from build123d import *

# Parameters (mm, degrees)
F0_W     = 56.3871189952
F0_H     = 33.6253512651
F1_DEPTH = 2
F2_W     = 51.7
F2_H     = 11.2356165416
F3_DEPTH = 15.62
F4_W     = 51.7
F4_H     = 15.62
F5_DEPTH = 1.5


# Not quite as in the source:
# - a feature of the source that left no trace in its solid (it failed there, or was rolled back) is left out


with BuildPart() as f1:
    # F0 (on Top) → F1 (new body)
    with BuildSketch(Plane.XY):
        with Locations((-6.0005225241, 2.1580690518)):
            Rectangle(F0_W, F0_H)
    extrude(amount=F1_DEPTH)

    # F2 (on face) → F3 (join)
    with BuildSketch(Plane.XY.offset(2)):
        with Locations((-5.8556830972, -9.0367983099)):
            Rectangle(F2_W, F2_H)
    extrude(amount=F3_DEPTH)

    # F4 (on face) → F5 (join)
    with BuildSketch(Plane.XZ.offset(14.6546065807)):
        with Locations((-5.8556830972, 9.81)):
            Rectangle(F4_W, F4_H)
    extrude(amount=F5_DEPTH)


solid = f1.part
Verification items for the finished model (mm, model axes). A direction names the side the tool comes from. Coordinates: 2 decimals unless noted, no trailing zeros. Order: outer loops, then holes, each group sorted by start corner. A loop starts at its lowest first (then second) coordinate and runs counter-clockwise, first axis right, second up. Notation, with made-up numbers: M -27,-2.75 L 21,-2.75 A5 cw 21,5.25 Z; hole C 15,-17 d6. An arc over 180 degrees is marked long. One line per item, written item: value. Start each with the question number.
Item 1: Sectioned sample at A-A (y = -13.5). Enter the section's corners in (x, z), then the cut area to 3 significant figures.
Item 2: Gauge pin test, flat ends, axial feed: pin 1 (1 mm diameter, centred on y = -7, z = 9.5, fed in from -X); pin 2 (1.6 mm diameter, centred on x = -8, y = -15.5, fed in from -Z); pin 3 (2 mm diameter, centred on x = 9, z = 11.5, fed in from +Y). Record the tip position at first contact, or that the pin passes through.
Item 3: Access from +Z, -Z, +X, -X, +Y, -Y to the whole of each face (thin tool, end or side, straight path). Record for faces 1 (the flat face through (19.994, -10, 10)), 2 (the flat face through (-6, -14.655, 1)), 3 (the flat face through (-31.706, -10, 10)), 4 (the flat face through (-6, -3.419, 10)), 5 (the flat face through (-34.194, 2, 1)).
Item 4: Sectioned sample at D-D (y = 4.5). Enter the section's corners in (x, z), then the cut area to 3 significant figures.
Item 5: Sectioned sample at C-C (z = 10.75). Enter the section's corners in (x, y), then the cut area to 3 significant figures.
Item 6: Sectioned sample at B-B (x = 11). Enter the section's corners in (y, z), then the cut area to 3 significant figures.
Item 7: Scan lines: probe 1 along X at (y, z) = (-10.5, 13); probe 2 along Z at (x, y) = (-9.5, 12); probe 3 along Y at (x, z) = (10, 12). Record each from-to range of solid material in increasing order.
Conclusion:
1. outline: M -34.19,0 L 22.19,0 L 22.19,2 L 19.99,2 L 19.99,17.62 L -31.71,17.62 L -31.71,2 L -34.19,2 Z
1. area: 920 mm^2
2. pin 1: stops at x = -31.71
2. pin 2: stops at z = 2
2. pin 3: stops at y = -3.42
3. face 1: +Z, +X, +Y, -Y
3. face 2: -Z, +X, -X, -Y
3. face 3: +Z, -X, +Y, -Y
3. face 4: +Z, +X, -X, +Y
3. face 5: +Z, -Z, -X, +Y, -Y
4. outline: M -34.19,0 L 22.19,0 L 22.19,2 L -34.19,2 Z
4. area: 113 mm^2
5. outline: M -31.71,-16.15 L 19.99,-16.15 L 19.99,-3.42 L -31.71,-3.42 Z
5. area: 658 mm^2
6. outline: M -16.15,2 L -14.65,2 L -14.65,0 L 18.97,0 L 18.97,2 L -3.42,2 L -3.42,17.62 L -16.15,17.62 Z
6. area: 266 mm^2
7. probe 1: x = -31.71 to 19.99
7. probe 2: z = 0 to 2
7. probe 3: y = -16.15 to -3.42
